Source: CAD feature listing. Evaluate the final solid. Frame: model axes, mm. Face numbers are marked on the shaded views. A direction names the side the tool comes from. Round coordinates to 2 decimals unless told otherwise and drop trailing zeros. Order: outer loops, then holes, each group sorted by start corner. A loop starts at its lowest first (then second) coordinate and runs counter-clockwise, first axis right, second up.
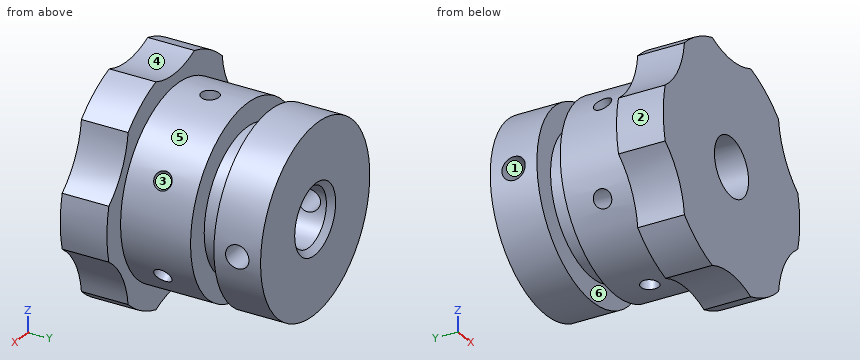
```python
from build123d import *

# Parameters (mm, degrees)
CUT_EXTRUDE1_REACH = 103.6
CUT_EXTRUDE2_REACH = 103.6
SKETCH3_R          = 15.875
CHAMFER1_SIZE      = 3.175
SKETCH4_R          = 6.35
CUT_EXTRUDE3_DEPTH = 50.8
SKETCH5_R          = 4.826
CUT_EXTRUDE4_DEPTH = 50.8
CIRPATTERN1_COUNT  = 6


with BuildPart() as part:
    # Sketch1 → Revolve1 (revolve)
    with BuildSketch(Plane.XY):
        Polygon((0, 0), (50.8, 0), (50.8, -25.4), (38.1, -25.4), (38.1, -38.1), (50.8, -38.1), (50.8, -76.2), (63.5, -76.2), (63.5, -101.6), (0, -101.6), align=None)
    revolve(axis=Axis((0, 0, 0), (0, -1, 0)))

    # Sketch2 → Cut-Extrude1 (cut, up to next)
    with BuildSketch(Plane.XZ.offset(101.6), mode=Mode.PRIVATE) as cut_extrude1_sk1:
        with BuildLine():
            ThreePointArc((-17.915510735, 60.9203125), (0, 57.15), (17.915510735, 60.9203125))
            ThreePointArc((17.915510735, 60.9203125), (0, 63.5), (-17.915510735, 60.9203125))
        make_face()
    cut_extrude1_tool1 = extrude(cut_extrude1_sk1.sketch, amount=-CUT_EXTRUDE1_REACH, mode=Mode.PRIVATE) & part.part
    add(cut_extrude1_tool1.solids().sort_by_distance((0, -101.6, 60.438615))[0], mode=Mode.SUBTRACT)
    # Sketch2 → Cut-Extrude1 (cut, up to next)
    with BuildSketch(Plane.XZ.offset(101.6), mode=Mode.PRIVATE) as cut_extrude1_sk2:
        with BuildLine():
            ThreePointArc((-43.800782864, 45.975443668), (-54.99261314, 31.75), (-61.716293599, 14.944868832))
            ThreePointArc((-61.716293599, 14.944868832), (-49.493351826, 28.575), (-43.800782864, 45.975443668))
        make_face()
    cut_extrude1_tool2 = extrude(cut_extrude1_sk2.sketch, amount=-CUT_EXTRUDE1_REACH, mode=Mode.PRIVATE) & part.part
    add(cut_extrude1_tool2.solids().sort_by_distance((-52.341376, -101.6, 30.219308))[0], mode=Mode.SUBTRACT)
    # Sketch2 → Cut-Extrude1 (cut, up to next)
    with BuildSketch(Plane.XZ.offset(101.6), mode=Mode.PRIVATE) as cut_extrude1_sk3:
        with BuildLine():
            ThreePointArc((43.800782864, 45.975443668), (49.493351826, 28.575), (61.716293599, 14.944868832))
            ThreePointArc((61.716293599, 14.944868832), (54.99261314, 31.75), (43.800782864, 45.975443668))
        make_face()
    cut_extrude1_tool3 = extrude(cut_extrude1_sk3.sketch, amount=-CUT_EXTRUDE1_REACH, mode=Mode.PRIVATE) & part.part
    add(cut_extrude1_tool3.solids().sort_by_distance((52.341376, -101.6, 30.219308))[0], mode=Mode.SUBTRACT)
    # Sketch2 → Cut-Extrude1 (cut, up to next)
    with BuildSketch(Plane.XZ.offset(101.6), mode=Mode.PRIVATE) as cut_extrude1_sk4:
        with BuildLine():
            ThreePointArc((61.716293599, -14.944868832), (49.493351826, -28.575), (43.800782864, -45.975443668))
            ThreePointArc((43.800782864, -45.975443668), (54.99261314, -31.75), (61.716293599, -14.944868832))
        make_face()
    cut_extrude1_tool4 = extrude(cut_extrude1_sk4.sketch, amount=-CUT_EXTRUDE1_REACH, mode=Mode.PRIVATE) & part.part
    add(cut_extrude1_tool4.solids().sort_by_distance((52.341376, -101.6, -30.219308))[0], mode=Mode.SUBTRACT)
    # Sketch2 → Cut-Extrude1 (cut, up to next)
    with BuildSketch(Plane.XZ.offset(101.6), mode=Mode.PRIVATE) as cut_extrude1_sk5:
        with BuildLine():
            ThreePointArc((17.915510735, -60.9203125), (0, -57.15), (-17.915510735, -60.9203125))
            ThreePointArc((-17.915510735, -60.9203125), (0, -63.5), (17.915510735, -60.9203125))
        make_face()
    cut_extrude1_tool5 = extrude(cut_extrude1_sk5.sketch, amount=-CUT_EXTRUDE1_REACH, mode=Mode.PRIVATE) & part.part
    add(cut_extrude1_tool5.solids().sort_by_distance((0, -101.6, -60.438615))[0], mode=Mode.SUBTRACT)
    # Sketch2 → Cut-Extrude1 (cut, up to next)
    with BuildSketch(Plane.XZ.offset(101.6), mode=Mode.PRIVATE) as cut_extrude1_sk6:
        with BuildLine():
            ThreePointArc((-43.800782864, -45.975443668), (-49.493351826, -28.575), (-61.716293599, -14.944868832))
            ThreePointArc((-61.716293599, -14.944868832), (-54.99261314, -31.75), (-43.800782864, -45.975443668))
        make_face()
    cut_extrude1_tool6 = extrude(cut_extrude1_sk6.sketch, amount=-CUT_EXTRUDE1_REACH, mode=Mode.PRIVATE) & part.part
    add(cut_extrude1_tool6.solids().sort_by_distance((-52.341376, -101.6, -30.219308))[0], mode=Mode.SUBTRACT)

    # Sketch3 → Cut-Extrude2 (cut, up to next)
    with BuildSketch(Plane(origin=(0, 0, 0), x_dir=(1, 0, 0), z_dir=(0, 1, 0)), mode=Mode.PRIVATE) as cut_extrude2_sk1:
        Circle(SKETCH3_R)
    cut_extrude2_tool1 = extrude(cut_extrude2_sk1.sketch, amount=-CUT_EXTRUDE2_REACH, mode=Mode.PRIVATE) & part.part
    add(cut_extrude2_tool1.solids().sort_by_distance((0, 0, 0))[0], mode=Mode.SUBTRACT)

    # Chamfer1
    chamfer1_edges = [part.edges().sort_by_distance(p)[0] for p in [
        (-15.875, 0, 0),
    ]]
    chamfer(chamfer1_edges, length=CHAMFER1_SIZE)

    # Sketch4 → Cut-Extrude3 (cut, symmetric)
    with BuildSketch(Plane(origin=(0, 0, 0), x_dir=(0, 0, -1), z_dir=(1, 0, 0))):
        with Locations((0, -12.7)):
            Circle(SKETCH4_R)
    extrude(amount=CUT_EXTRUDE3_DEPTH, both=True, mode=Mode.SUBTRACT)

    # Sketch5 → Cut-Extrude4 (cut, symmetric)
    with BuildSketch(Plane.XY):
        with Locations((0, -57.15)):
            Circle(SKETCH5_R)
    cut_extrude4 = extrude(amount=CUT_EXTRUDE4_DEPTH, both=True, mode=Mode.SUBTRACT)

    # CirPattern1: Cut-Extrude4 ×6 about axis
    cirpattern1_axis = Axis((0, -38.1, 0), (0, 1, 0))
    for i in range(1, CIRPATTERN1_COUNT):
        add(cut_extrude4.rotate(cirpattern1_axis, i * 360 / CIRPATTERN1_COUNT), mode=Mode.SUBTRACT)


solid = part.part
```
1. Section A-A on y = -92. Return loops of the section in (x, z) (3 decimals).
2. Access query for the marked faces 4, 5 and 6. Directions: +Z, -Z, +X, -X, +Y, -Y. A direction counts if a zero-diameter tool reaches every point of the face in a straight line with its end or side. Return the directions, or none.
3. First-contact query: pin 1 (6 mm diameter, centred on y = -39, z = -42, fed in from +X); pin 2 (12.5 mm diameter, centred on x = 0, y = -57.15, fed in from -Z); pin 3 (4 mm diameter, centred on x = 24.5, y = -83, fed in from +Z); pin 4 (19 mm diameter, centred on x = 0, z = 0, fed in from -Y). Flat tips, straight axial feed; report the tip coordinate or a pass-through.
4. Pull-direction query (X, two-part tool) for the marked faces 1, 2 and 3; classes: released by +X, released by -X, zero draft, split by the parting line, or undercut.
5. Section D-D on y = -12.7. Return loops of the section in (x, z) (3 decimals), plus the area to 3 significant figures.
6. Section B-B on x = 0. State how many separate pieces and enclosed holes the cut face has, plus the area to 3 significant figures.
7. Line query: line 1 along Y through (x, z) = (10.5, 48.5); line 2 along Y through (x, z) = (-49, 4.5); line 3 along Y through (x, z) = (0, 28). Output: solid intervals per line, ascending.
Result:
1. outline: (-61.716, -14.945) arc R44.45 cw to (-43.801, -45.975) arc R63.5 ccw to (-17.916, -60.92) arc R44.45 cw to (17.916, -60.92) arc R63.5 ccw to (43.801, -45.975) arc R44.45 cw to (61.716, -14.945) arc R63.5 ccw to (61.716, 14.945) arc R44.45 cw to (43.801, 45.975) arc R63.5 ccw to (17.916, 60.92) arc R44.45 cw to (-17.916, 60.92) arc R63.5 ccw to (-43.801, 45.975) arc R44.45 cw to (-61.716, 14.945) arc R63.5 ccw to start; hole circle Ø31.75 at (0, 0)
2. face 4: +Z, +Y, -Y
2. face 5: +Y
2. face 6: none
3. pin 1: stops at x = 32.55
3. pin 2: stops at z = -50.8
3. pin 3: stops at z = 59.38
3. pin 4: passes through
4. face 1: zero draft
4. face 2: released by -X
4. face 3: undercut
5. outline: (-50.402, -6.35) arc R50.8 ccw to (50.402, -6.35) - (14.55, -6.35) arc R15.875 cw to (-14.55, -6.35) - close; (-50.402, 6.35) - (-14.55, 6.35) arc R15.875 cw to (14.55, 6.35) - (50.402, 6.35) arc R50.8 ccw to start
5. area: 6,420 mm2
6. separate pieces: 4
6. enclosed holes: 0
6. area: 6,410 mm2
7. line 1: y = -101.6 to -38.1, -25.4 to 0
7. line 2: y = -101.6 to -38.1, -25.4 to -17.18, -8.22 to 0
7. line 3: y = -101.6 to -61.98, -52.32 to 0
